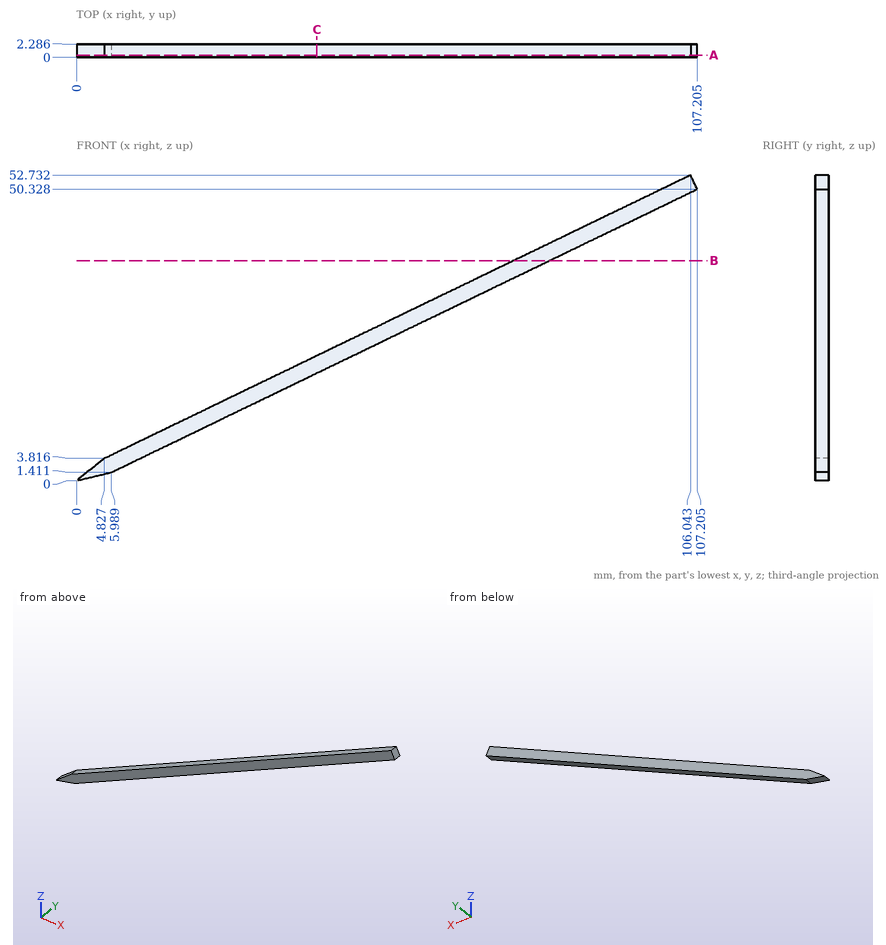
Print and shaded views of the part. All mm, measured from the part's lowest x, y and z. Give positions to 0.01 mm unless a question says otherwise; leave off trailing zeros. Loops run counter-clockwise (first coordinate to the right, second up) from the corner with the lowest first, then second, coordinate; pieces in that order, holes last.
1) Wall check: line 1 (X direction, y = 0.45, z = 22.5) (1 decimal); line 2 (Z direction, x = 53, y = 0.4); line 3 (X direction, y = 2.1, z = 45.5) (1 decimal). Give the ranges that are in metal, low to high.
2) Saw through at B-B (z = 38). Write the cut outline in (x, y).
3) Saw through at C-C (x = 41.5). Write the cut outline in (y, z).
4) Flat gauge pin, fed straight in: pin 1 Ø1 at (y, z) = (0, 36.5) entering from -X. Where does the tip first touch, or does it go through?
5) Saw through at A-A (y = 0.35). Write the cut outline in (x, z) (1 decimal).
Answer block:
1. line 1: x = 43.5 to 49.6
1. line 2: z = 24.13 to 27.1
1. line 3: x = 91.1 to 97.2
2. outline: (75.56, 0) - (81.7, 0) - (81.7, 2.29) - (75.56, 2.29) - close
3. outline: (0, 18.57) - (2.29, 18.57) - (2.29, 21.54) - (0, 21.54) - close
4. pin 1: stops at x = 71.42
5. outline: (0, 0) - (6, 1.4) - (107.2, 50.3) - (106, 52.7) - (4.8, 3.8) - close
